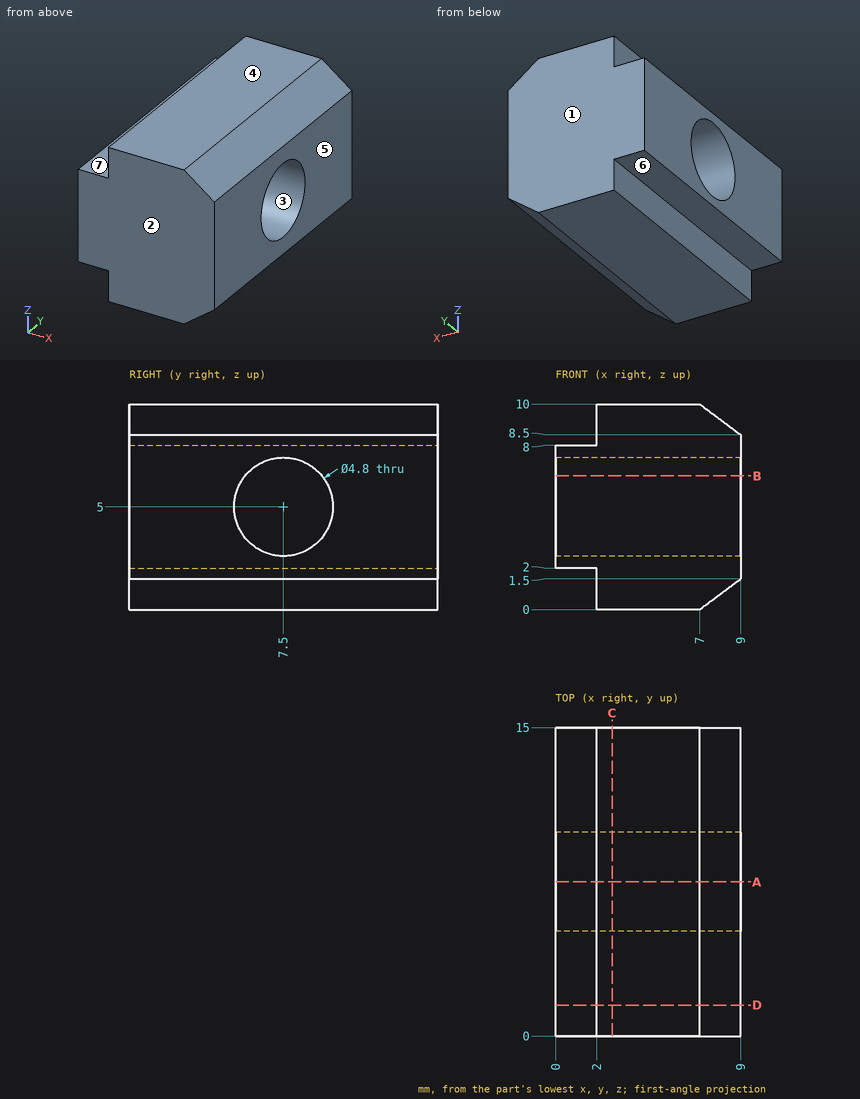
Geometry: see drawing. Coordinates: mm, zero at the bounding-box minimum. A direction names the side the tool comes from. Coordinates: 2 decimals unless noted, no trailing zeros. Write each loop counter-clockwise with the first axis right and the second up, starting at its lowest first coordinate (ties: lowest second). Pieces come first, ordered by that corner, then holes. Notation, with made-up numbers: M 41,58 L 62,58 A7 cw 62,62 Z; hole C 57,-25 d7. An arc over 180 degrees is marked long. Use CSV: the item, a comma, the result in double quotes. Start each with the question number.
1. Mould query, pull axis Y, two halves, no side actions, for the marked faces 1, 2, 3 and 4. Classes: pulls with the +Y half, pulls with the -Y half, needs draft (parallel to the pull), parting line crosses it, or undercut.
2. Cut plane C-C on x = 2.75. Return the cut outline in (y, z).
3. First-contact query: P1, Ø2, axis at x = 0.5, y = 5.5, coming from the +Z side; P2, Ø1, axis at y = 4.5, z = 9, coming from the -X side; P3, Ø1, axis at x = 0.5, y = 10.5, coming from the -Z side. Flat tips, straight axial feed; report the tip coordinate or a pass-through.
4. Reachability of the marked faces 5, 6 and 7 from +Z, -Z, +X, -X, +Y, -Y: full face, straight path, thin tool, end or side. Return the list, or none.
5. Ray query, probe 1 along Y at (x, z) = (6.5, 5); probe 2 along Y at (x, z) = (3, 3.75); probe 3 along Z at (x, y) = (7.5, 6) (1 decimal). Return the intervals inside material, ascending.
6. Cut plane B-B on z = 6.5. Return the cut outline in (x, y).
7. Cut plane D-D on y = 1.5. Return the cut outline in (x, z).
8. Cut plane A-A on y = 7.5. Return the cut outline in (x, z), plus the area to 3 significant figures.
Entries:
1,face 1,"pulls with the +Y half"
1,face 2,"pulls with the -Y half"
1,face 3,"undercut"
1,face 4,"needs draft"
2,outline,"M 0,0 L 15,0 L 15,10 L 0,10 Z; hole C 7.5,5 d4.8"
3,P1,"z = 8"
3,P2,"x = 2"
3,P3,"z = 2"
4,face 5,"+Z, -Z, +X, +Y, -Y"
4,face 6,"-Z, -X, +Y, -Y"
4,face 7,"+Z, -X, +Y, -Y"
5,probe 1,"0 to 5.1, 9.9 to 15"
5,probe 2,"0 to 5.45, 9.55 to 15"
5,probe 3,"0.4 to 3.1, 6.9 to 9.6"
6,outline,"M 0,0 L 9,0 L 9,5.63 L 0,5.63 Z; M 0,9.37 L 9,9.37 L 9,15 L 0,15 Z"
7,outline,"M 0,2 L 2,2 L 2,0 L 7,0 L 9,1.5 L 9,8.5 L 7,10 L 2,10 L 2,8 L 0,8 Z"
8,outline,"M 0,2 L 2,2 L 2,0 L 7,0 L 9,1.5 L 9,2.6 L 0,2.6 Z; M 0,7.4 L 9,7.4 L 9,8.5 L 7,10 L 2,10 L 2,8 L 0,8 Z"
8,area,"35.8 mm²"
